from build123d import *

# Parameters (mm, degrees)
F0_R      = 50.8
F0_R_2    = 47.625
F1_DEPTH  = 482.6
F4_DEPTH  = 508
F5_W      = 55.5464364588
F5_H      = 92.0769795775
F6_DEPTH  = 508
F7_W      = 106.5891161561
F7_H      = 48.0401627719
F8_DEPTH  = 101.6
F9_W      = 58.4661662579
F9_H      = 32.7058173716
F10_DEPTH = 82.55


# Not quite as in the source:
# - the program builds the solid bodies; features that only make, move or delete a surface that nothing else refers to are left out


with BuildPart() as f1:
    # F0 (on Right) → F1 (new body)
    with BuildSketch(Plane.YZ):
        Circle(F0_R)
        Circle(F0_R_2, mode=Mode.SUBTRACT)
    extrude(amount=F1_DEPTH)

    # F3 (on Right) → F4 (cut)
    with BuildSketch(Plane.YZ):
        Polygon((0, 91.0463854671), (0, 0), (0, -77.0941823721), (61.9923658669, -77.0941823721), (61.9923658669, 91.0463854671), align=None)
    extrude(amount=F4_DEPTH, mode=Mode.SUBTRACT)

    # F5 (on Right) → F6 (cut)
    with BuildSketch(Plane.YZ):
        with Locations((27.7732182294, 46.0384897888)):
            Rectangle(F5_W, F5_H)
    extrude(amount=F6_DEPTH, mode=Mode.SUBTRACT)

    # F7 (on Top) → F8 (cut)
    with BuildSketch(Plane.XY):
        with Locations((53.2945580781, 24.020081386)):
            Rectangle(F7_W, F7_H)
    extrude(amount=F8_DEPTH, mode=Mode.SUBTRACT)

    # F9 (on Top) → F10 (cut)
    with BuildSketch(Plane.XY):
        with Locations((77.5640532374, 16.3529086858)):
            Rectangle(F9_W, F9_H)
    extrude(amount=F10_DEPTH, mode=Mode.SUBTRACT)


solid = f1.part
Design review of the part built by this model. Coordinates are the model's own, in mm. Coordinates: 2 decimals unless noted, no trailing zeros. Order: outer loops, then holes, each group sorted by start corner. A loop starts at its lowest first (then second) coordinate and runs counter-clockwise, first axis right, second up. Notation, with made-up numbers: (-5.5, 19) -> (32.5, 19) arc R21 cw to (32.5, 40) -> close; hole circle Ø6 at (57.5, 31.5). An arc over 180 degrees is marked (long way). One line per item, written item: value.
1) We need section A-A, the plane y = -15.5. Give the boundary of the cut face in (x, z).
Output values:
outline: (0, -48.38) -> (482.6, -48.38) -> (482.6, -45.03) -> (0, -45.03) -> close; (0, 45.03) -> (482.6, 45.03) -> (482.6, 48.38) -> (0, 48.38) -> close
2) To check wall thickness, follow probe 1 along Z at (x, y) = (353, -3); probe 2 along Z at (x, y) = (120.5, -20); probe 3 along Y at (x, z) = (338, 35.5). State the ranges of each line that lie inside material, in increasing order. Write a range as [from, to].
Output values:
probe 1: z = [-50.71, -47.53], [47.53, 50.71]
probe 2: z = [-46.7, -43.22], [43.22, 46.7]
probe 3: y = [-36.34, -31.75]
3) We need section D-D, the plane x = 425. Give the boundary of the cut face in (y, z) (3 decimals), then the cut area to 3 significant figures.
Output values:
outline: (0, -50.8) -> (0, -47.625) arc R47.625 cw to (0, 47.625) -> (0, 50.8) arc R50.8 ccw to start
area: 491 mm2
4) Clearance check with flat-ended pins moving along their axes: P1, Ø4, axis at x = 154.5, y = -38.5, coming from the -Z side; P2, Ø1.5, axis at x = 372, z = -18.5, coming from the -Y side; P3, Ø1.5, axis at x = 414, y = -39.5, coming from the -Z side. State where each tip first meets the part, or that it passes through.
Output values:
P1: stops at z = -35.33
P2: stops at y = -47.6
P3: stops at z = -32.85
5) Draft analysis for pull direction Z (two halves, no side actions). For faces 1 (the face through (0, -48, 0)), 2 (the face through (237.922, -50.788, 1.117)), 3 (the face through (237.922, -47.613, 1.047)), state which applies: +Z half, -Z half, draft (parallel to the pull), parting line (faces both ways), or undercut.
Output values:
face 1: draft
face 2: parting line
face 3: undercut
6) We need section C-C, the plane y = -37. Give the boundary of the cut face in (x, z).
Output values:
outline: (0, -34.81) -> (482.6, -34.81) -> (482.6, -29.99) -> (0, -29.99) -> close; (0, 29.99) -> (482.6, 29.99) -> (482.6, 34.81) -> (0, 34.81) -> close
7) We need section B-B, the plane z = 0. Give the boundary of the cut face in (x, y) (3 decimals).
Output values:
outline: (0, -50.8) -> (482.6, -50.8) -> (482.6, -47.625) -> (0, -47.625) -> close
